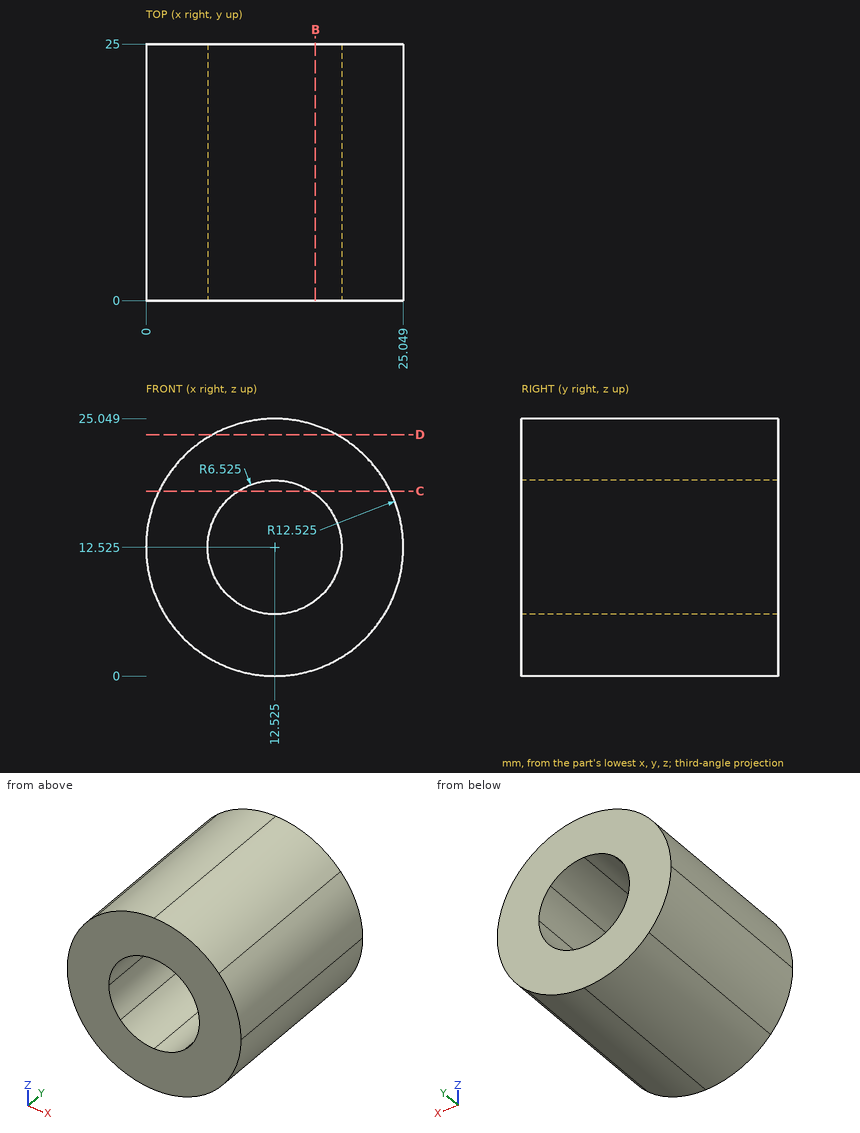
Verification items for this drawing (mm, ordinates from the low corner). Give positions to 0.01 mm unless a question says otherwise; leave off trailing zeros. Write each loop counter-clockwise with the first axis right and the second up, starting at its lowest first coordinate (ties: lowest second). Pieces come first, ordered by that corner, then holes.
1) Section check B-B, the plane x = 16.5. Record the boundary of the cut face in (y, z).
2) Section check C-C, the plane z = 18. Record the boundary of the cut face in (x, y), and give its area (3 significant figures).
3) Section check D-D, the plane z = 23.5. Record the boundary of the cut face in (x, y), and give its area (3 significant figures).
4) Material ranges on L1, parallel to X at y = 5.5, z = 14.75; L2, parallel to X at y = 9.75, z = 18.5 (1 decimal); L3, parallel to Z at x = 8.5, y = 19.75 (1 decimal), recorded low to high.
5) Gauge pin test, flat ends, axial feed: pin 1 (1.5 mm diameter, centred on x = 20.5, y = 11.5, fed in from -Z) (1 decimal); pin 2 (1.5 mm diameter, centred on y = 12, z = 4, fed in from -X) (1 decimal). Record the tip position at first contact, or that the pin passes through.
Computed:
1. outline: (0, 0.65) - (25, 0.65) - (25, 7.35) - (0, 7.35) - close; (0, 17.7) - (25, 17.7) - (25, 24.4) - (0, 24.4) - close
2. outline: (1.26, 0) - (8.98, 0) - (8.98, 25) - (1.26, 25) - close; (16.07, 0) - (23.79, 0) - (23.79, 25) - (16.07, 25) - close
2. area: 386 mm2
3. outline: (6.49, 0) - (18.56, 0) - (18.56, 25) - (6.49, 25) - close
3. area: 302 mm2
4. L1: x = 0.2 to 6.39, 18.66 to 24.85
4. L2: x = 1.5 to 9.9, 15.1 to 23.5
4. L3: z = 0.7 to 7.4, 17.7 to 24.4
5. pin 1: stops at z = 2.3
5. pin 2: stops at x = 2.7
